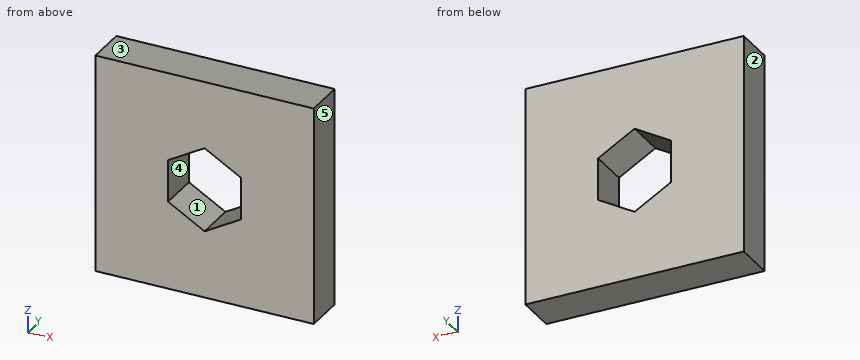
Autodesk Inventor part; units mm, degrees
ref_plane "YZ Plane" through (0, 0, 0) normal (1, 0, 0) x (0, 1, 0)
ref_plane "XZ Plane" through (0, 0, 0) normal (0, 1, 0) x (-1, 0, 0)
ref_plane "XY Plane" through (0, 0, 0) normal (0, 0, 1) x (1, 0, 0)
sketch "Sketch1" plane through (0, 0, 0) normal (0, 1, 0) x (-1, 0, 0)
  line L0 (7.9861, 7.7649) -> (7.9861, -43.0351)
  line L1 (7.9861, -43.0351) -> (-42.8139, -43.0351)
  line L2 (-42.8139, -43.0351) -> (-42.8139, 7.7649)
  line L3 (-42.8139, 7.7649) -> (7.9861, 7.7649)
  line L4 (-17.4139, -27.4351) -> (-25.901, -22.5351)
  line L5 (-25.901, -22.5351) -> (-25.901, -12.7351)
  line L6 (-25.901, -12.7351) -> (-17.4139, -7.8351)
  line L7 (-17.4139, -7.8351) -> (-8.9269, -12.7351)
  line L8 (-8.9269, -12.7351) -> (-8.9269, -22.5351)
  line L9 (-8.9269, -22.5351) -> (-17.4139, -27.4351)
  point P0 (0, 0)
  point P1 (-17.4139, -17.6351)
  point P2 (-21.6575, -24.9851)
  point P3 (-13.1704, -10.2851)
  dimension "d0" = 50.8
  dimension "d1" = 50.8
  dimension "d2" = 14.7
extrude "Extrusion1" add sketch "Sketch1" along normal blind 9.525
properties part number "Hex Box +2mm"
Work out the finished part from the listing and answer in its coordinate system (mm). Face numbers are marked on the shaded views. A direction names the side the tool comes from. Give positions to 0.01 mm unless a question says otherwise; leave off trailing zeros. Order: outer loops, then holes, each group sorted by start corner. A loop starts at its lowest first (then second) coordinate and runs counter-clockwise, first axis right, second up.
1. Section A-A, the plane y = 6.5 is taken. Determine the outline of the cut face in (x, z).
Result sheet:
outline: (-7.99, -43.04) - (42.81, -43.04) - (42.81, 7.76) - (-7.99, 7.76) - close; hole (8.93, -22.54) - (17.41, -27.44) - (25.9, -22.54) - (25.9, -12.74) - (17.41, -7.84) - (8.93, -12.74) - close
2. Straight lines are drawn through the part: L1, parallel to X at y = 3.75, z = -14; L2, parallel to Z at x = 21, y = 5.25; L3, parallel to X at y = 7.75, z = -25. For each, find the intervals that lie inside material, in ascending order.
Result sheet:
L1: x = -7.99 to 8.93, 25.9 to 42.81
L2: z = -43.04 to -25.36, -9.91 to 7.76
L3: x = -7.99 to 13.2, 21.63 to 42.81
3. Section B-B, the plane z = -20.5 is taken. Determine the outline of the cut face in (x, y) (3 decimals), and give its area (3 significant figures).
Result sheet:
outline: (-7.986, 0) - (8.927, 0) - (8.927, 9.525) - (-7.986, 9.525) - close; (25.901, 0) - (42.814, 0) - (42.814, 9.525) - (25.901, 9.525) - close
area: 322 mm2
4. Section C-C, the plane x = 23 is taken. Determine the outline of the cut face in (y, z) (3 decimals), and give its area (3 significant figures).
Result sheet:
outline: (0, -43.035) - (9.525, -43.035) - (9.525, -24.21) - (0, -24.21) - close; (0, -11.06) - (9.525, -11.06) - (9.525, 7.765) - (0, 7.765) - close
area: 359 mm2
5. For the marked faces 1 and 2, determine the directions among +Z, -Z, +X, -X, +Y, -Y from which every point of the face is accessible in a straight line to the end or side of a thin tool.
Result sheet:
face 1: +Y, -Y
face 2: +Z, -Z, -X, +Y, -Y
6. The mould has two halves that part along X. Classify the marked faces 3, 4 and 5: released by +X, released by -X, zero draft, split by the parting line, or undercut.
Result sheet:
face 3: zero draft
face 4: undercut
face 5: released by +X
